from build123d import *

# Parameters (mm, degrees)
EXTRUDE_1_DEPTH     = 1
CHAMFER_1_SIZE      = 0.6
SKETCH_2_W          = 6
SKETCH_2_H          = 6
EXTRUDE_2_DEPTH     = 3
SKETCH_3_R          = 1.2
CUT_EXTRUDE_1_DEPTH = 5
SKETCH_4_R          = 2.05
CUT_EXTRUDE_2_DEPTH = 2
FILLET_1_R          = 2
CUT_EXTRUDE_3_DEPTH = 5
FILLET_2_R          = 0.4
FILLET_3_R          = 1.2
CHAMFER_2_SIZE      = 0.4


with BuildPart() as part:
    # 草图1 → 凸台-拉伸1 (new body)
    with BuildSketch(Plane(origin=(0, 0, 0), x_dir=(1, 0, 0), z_dir=(0, 1, 0))):
        Polygon((0, 0), (44, 44), (44, 62), (29, 77), (18, 66), (13.757359313, 66), (-2.3, 49.942640687), (-2.3, 45.7), (-10, 38), (-10, 10), align=None)
    extrude(amount=EXTRUDE_1_DEPTH)

    # 倒角1
    chamfer_1_edges = [part.edges().sort_by_distance(p)[0] for p in [
        (44, 1, -53),
        (36.5, 1, -69.5),
        (23.5, 1, -71.5),
        (15.878679656, 1, -66),
        (5.728679656, 1, -57.971320344),
        (-2.3, 1, -47.821320344),
        (-6.15, 1, -41.85),
        (-10, 1, -24),
        (-5, 1, -5),
        (22, 1, -22),
    ]]
    chamfer(chamfer_1_edges, length=CHAMFER_1_SIZE)

    # 草图2 → 凸台-拉伸2 (add)
    with BuildSketch(Plane.XZ):
        with Locations((-7, -24)):
            Rectangle(SKETCH_2_W, SKETCH_2_H)
        with Locations((25, -47)):
            Rectangle(SKETCH_2_W, SKETCH_2_H)
    extrude(amount=EXTRUDE_2_DEPTH)

    # 草图3 → 切除-拉伸1 (cut, through all)
    with BuildSketch(Plane(origin=(0, -3, 0), x_dir=(-1, 0, 0), z_dir=(0, -1, 0))):
        with Locations((6.9, 24)):
            Circle(SKETCH_3_R)
        with Locations((-25, 46.9)):
            Circle(SKETCH_3_R)
    extrude(amount=-CUT_EXTRUDE_1_DEPTH, mode=Mode.SUBTRACT)

    # 草图4 → 切除-拉伸2 (cut)
    with BuildSketch(Plane(origin=(0, 1, 0), x_dir=(1, 0, 0), z_dir=(0, 1, 0))):
        with Locations((-6.9, 24)):
            Circle(SKETCH_4_R)
        with Locations((25, 46.9)):
            Circle(SKETCH_4_R)
    extrude(amount=-CUT_EXTRUDE_2_DEPTH, mode=Mode.SUBTRACT)

    # 圆角1
    fillet_1_edges = [part.edges().sort_by_distance(p)[0] for p in [
        (-4, -1.5, -27),
        (-4, -1.5, -21),
        (22, -1.5, -44),
        (22, -1.5, -50),
        (28, -1.5, -50),
        (28, -1.5, -44),
    ]]
    fillet(fillet_1_edges, radius=FILLET_1_R)

    # 草图5 → 切除-拉伸3 (cut, through all)
    with BuildSketch(Plane(origin=(0, 1, 0), x_dir=(1, 0, 0), z_dir=(0, 1, 0))):
        Polygon((14.352847127, 24.4), (15.5, 26.038304089), (4.851023424, 33.494797761), (3.703870552, 31.856493673), align=None)
        Polygon((14.352847127, 31.4), (3.444218368, 39.038304089), (14.352847127, 46.676608177), (15.5, 45.038304089), (6.93111196, 39.038304089), (15.5, 33.038304089), align=None)
    extrude(amount=-CUT_EXTRUDE_3_DEPTH, mode=Mode.SUBTRACT)

    # 圆角2
    fillet_2_edges = [part.edges().sort_by_distance(p)[0] for p in [
        (14.352847127, 0.5, -24.4),
        (3.703870552, 0.5, -31.856493673),
        (4.851023424, 0.5, -33.494797761),
        (15.5, 0.5, -26.038304089),
        (15.5, 0.5, -33.038304089),
        (14.352847127, 0.5, -31.4),
        (14.352847127, 0.5, -46.676608177),
        (15.5, 0.5, -45.038304089),
        (6.93111196, 0.5, -39.038304089),
    ]]
    fillet(fillet_2_edges, radius=FILLET_2_R)

    # 圆角3
    fillet_3_edges = [part.edges().sort_by_distance(p)[0] for p in [
        (3.444218368, 0.5, -39.038304089),
    ]]
    fillet(fillet_3_edges, radius=FILLET_3_R)

    # 倒角2
    chamfer_2_edges = [part.edges().sort_by_distance(p)[0] for p in [
        (11.285699643, 1, -42.08741921),
        (9.028358839, 1, -28.128246836),
        (4.277446988, 1, -32.675645717),
        (10.175511712, 1, -29.766550925),
        (14.926423564, 1, -25.219152044),
        (14.926423564, 1, -32.219152044),
        (9.436624555, 1, -43.234232072),
        (14.926423564, 1, -45.857456133),
        (11.285699643, 1, -35.989188967),
        (7.228490678, 1, -39.038304089),
        (14.324076155, 1, -46.513439886),
        (15.336831709, 1, -45.067075061),
        (15.336831709, 1, -33.009533116),
        (14.324076155, 1, -31.563168291),
        (15.336831709, 1, -26.009533116),
        (14.324076155, 1, -24.563168291),
        (4.879794396, 1, -33.33162947),
        (3.867038843, 1, -31.885264645),
        (9.436624555, 1, -34.842376105),
        (4.336354523, 1, -39.038304089),
    ]]
    chamfer(chamfer_2_edges, length=CHAMFER_2_SIZE)


solid = part.part
The model under review builds one solid part; all positions refer to its coordinate system, in mm. A direction names the side the tool comes from. Give positions to 0.01 mm unless a question says otherwise; leave off trailing zeros. Loops run counter-clockwise (first coordinate to the right, second up) from the corner with the lowest first, then second, coordinate; pieces in that order, holes last. Notation, with made-up numbers: (35, 30) -> (81, 30) arc R38 ccw to (81, 68) -> close; hole circle Ø7 at (36, 25). An arc over 180 degrees is marked (long way). Answer as a JSON object with one key per item and string values. Group by question number.
Q1. Take a section at B-B (z = -28). Write out the cut boundary in (x, y).
Q2. Insertion check: pin 1 (1.6 mm diameter, centred on x = 25.5, y = -1, fed in from -Z); pin 2 (1.5 mm diameter, centred on y = -0.5, z = -33, fed in from +X); pin 3 (0.6 mm diameter, centred on y = -2, z = -24, fed in from +X); pin 4 (1.9 mm diameter, centred on x = -6.9, z = -24, fed in from +Y). Each pin has a flat end and moves straight along its axis. Give the tip position at first contact, or say it passes through.
Q3. Wall thickness on line 1 along Z through (x, y) = (-6.9, -0.2); line 2 along Z through (x, y) = (7.5, 0.8); line 3 along X through (y, z) = (-0.05, -46.9): over which ranges is each line inside the solid? List them lowest first.
Q4. Take a section at C-C (x = 32.5). Write out the cut boundary in (y, z).
Q5. Take a section at D-D (x = 25). Write out the cut boundary in (y, z), plus the area to 3 significant figures.
Q6. Tool access review of faces 5 (the cylindrical face through (22.57, -1.52, -44.6)), 6 (the cylindrical face through (27.43, -1.52, -49.4)), 7 (the flat face through (28, -1, -47)), 8 (the flat face through (11.35, 0.8, -36.19)): name each direction out of +Z, -Z, +X, -X, +Y, -Y from which nothing blocks a thin tool from reaching the whole face with its end or side.
Q7. Take a section at A-A (x = -6.9). Write out the cut boundary in (y, z).
Q8. Draft analysis for pull direction Z (two halves, no side actions). For faces 1 (the flat face through (17, 1, -39)), 2 (the flat face through (9.37, 0.3, -43.19)), 3 (the cylindrical face through (27.4, -1.52, -44.57)), 4 (the flat face through (23.6, 0.2, -71.6)), state which applies: pulls with the +Z half, pulls with the -Z half, needs draft (parallel to the pull), parting line crosses it, or undercut.
Answer below:
{
 "1": {"outline": "(-10, 0) -> (9.21, 0) -> (9.21, 0.6) -> (8.51, 1) -> (-9.4, 1) -> (-10, 0.4) -> close; (12.7, 0) -> (28, 0) -> (28, 0.4) -> (27.15, 1) -> (13.4, 1) -> (12.7, 0.6) -> close"},
 "2": {"pin 1": "stops at z = -50", "pin 2": "stops at x = 33.56", "pin 3": "stops at x = -4", "pin 4": "passes through"},
 "3": {"line 1": "z = -27 to -26.05, -21.95 to -21", "line 2": "z = -59.18 to -42.12, -39.19 to -38.89, -35.95 to -31.88, -28.95 to -8.07", "line 3": "x = 22 to 22.95, 27.05 to 28"},
 "4": {"outline": "(0, -73.5) -> (0.4, -73.5) -> (1, -72.65) -> (1, -33.35) -> (0.4, -32.5) -> (0, -32.5) -> close"},
 "5": {"outline": "(-3, -50) -> (0, -50) -> (0, -73) -> (0.4, -73) -> (1, -72.15) -> (1, -48.95) -> (-1, -48.95) -> (-1, -48.1) -> (-3, -48.1) -> close; (-3, -45.7) -> (-1, -45.7) -> (-1, -44.85) -> (1, -44.85) -> (1, -25.85) -> (0.4, -25) -> (0, -25) -> (0, -44) -> (-3, -44) -> close", "area": "52.5 mm2"},
 "6": {"face 5": "+Z, -X, -Y", "face 6": "-Z, +X, -Y", "face 7": "+Z, -Z, +X, -Y", "face 8": "+Y"},
 "7": {"outline": "(-3, -27) -> (0, -27) -> (0, -41.1) -> (0.4, -41.1) -> (1, -40.25) -> (1, -26.05) -> (-1, -26.05) -> (-1, -25.2) -> (-3, -25.2) -> close; (-3, -22.8) -> (-1, -22.8) -> (-1, -21.95) -> (1, -21.95) -> (1, -7.75) -> (0.4, -6.9) -> (0, -6.9) -> (0, -21) -> (-3, -21) -> close"},
 "8": {"face 1": "needs draft", "face 2": "undercut", "face 3": "pulls with the +Z half", "face 4": "pulls with the -Z half"}
}
